Work out the finished part from the listing and answer in its coordinate system (mm). Round coordinates to 2 decimals unless told otherwise and drop trailing zeros. Order: outer loops, then holes, each group sorted by start corner. A loop starts at its lowest first (then second) coordinate and runs counter-clockwise, first axis right, second up. Notation, with made-up numbers: (13, 53.25) -> (62, 53.25) arc R23 ccw to (62, 87.25) -> close; hole circle Ø11 at (-22, 31). An arc over 180 degrees is marked (long way). Use a Markdown table: item, result. Add a question column.
Item 1: Find the intervals of material crossed by L1, parallel to Y at x = 0, z = 1.2; L2, parallel to X at y = -109, z = 1.55; L3, parallel to Y at x = 1, z = 0.3, in increasing order. Write a range as [from, to].
Item 2: A cutting plane is placed at C-C, the plane z = 0.9. Determine the outline of the cut face in (x, y), plus the area to 3 significant figures.
Item 3: A cutting plane is placed at B-B, the plane y = 109. Determine the outline of the cut face in (x, z).
Item 4: For a pull along Y with two mould halves and no side action, classify faces 1 (the cylindrical face through (0.521, -112.966, 0.986)), 2 (the flat face through (0, 2, 2)) as +Y half, -Y half, draft (parallel to the pull), parting line (faces both ways), or undercut.
Item 5: A cutting plane is placed at A-A, the plane x = 0. Determine the outline of the cut face in (y, z), plus the area to 3 significant figures.
from build123d import *

# Parameters (mm, degrees)
SKETCH1_R           = 4
BOSS_EXTRUDE1_DEPTH = 2


with BuildPart() as part:
    # Sketch1 → Boss-Extrude1 (new body)
    with BuildSketch(Plane.XY):
        Polygon((3.5, 121.5), (12.5, 121.5), (12.5, -121.5), (3.5, -121.5), (0, -121.5), (-12.5, -121.5), (-12.5, -115.487492178), (-12.5, -105.5), (-12.5, 112.5), (-12.5, 121.482064427), (-12.5, 121.5), (0, 121.5), align=None)
        with Locations((0, 109)):
            Circle(SKETCH1_R, mode=Mode.SUBTRACT)
        with Locations(Location((0, -109, 0), (0, 0, 180))):
            Circle(SKETCH1_R, mode=Mode.SUBTRACT)
    extrude(amount=BOSS_EXTRUDE1_DEPTH)


solid = part.part
Reported:
| question | item | result |
|---|---|---|
| 1 | L1 | [-121.5, -113], [-105, 105], [113, 121.5] |
| 1 | L2 | [-12.5, -4], [4, 12.5] |
| 1 | L3 | [-121.5, -112.87], [-105.13, 105.13], [112.87, 121.5] |
| 2 | outline | (-12.5, -121.5) -> (12.5, -121.5) -> (12.5, 121.5) -> (-12.5, 121.5) -> close; hole circle Ø8 at (0, -109); hole circle Ø8 at (0, 109) |
| 2 | area | 5,970 mm² |
| 3 | outline | (-12.5, 0) -> (-4, 0) -> (-4, 2) -> (-12.5, 2) -> close; (4, 0) -> (12.5, 0) -> (12.5, 2) -> (4, 2) -> close |
| 4 | face 1 | undercut |
| 4 | face 2 | draft |
| 5 | outline | (-121.5, 0) -> (-113, 0) -> (-113, 2) -> (-121.5, 2) -> close; (-105, 0) -> (105, 0) -> (105, 2) -> (-105, 2) -> close; (113, 0) -> (121.5, 0) -> (121.5, 2) -> (113, 2) -> close |
| 5 | area | 454 mm² |
